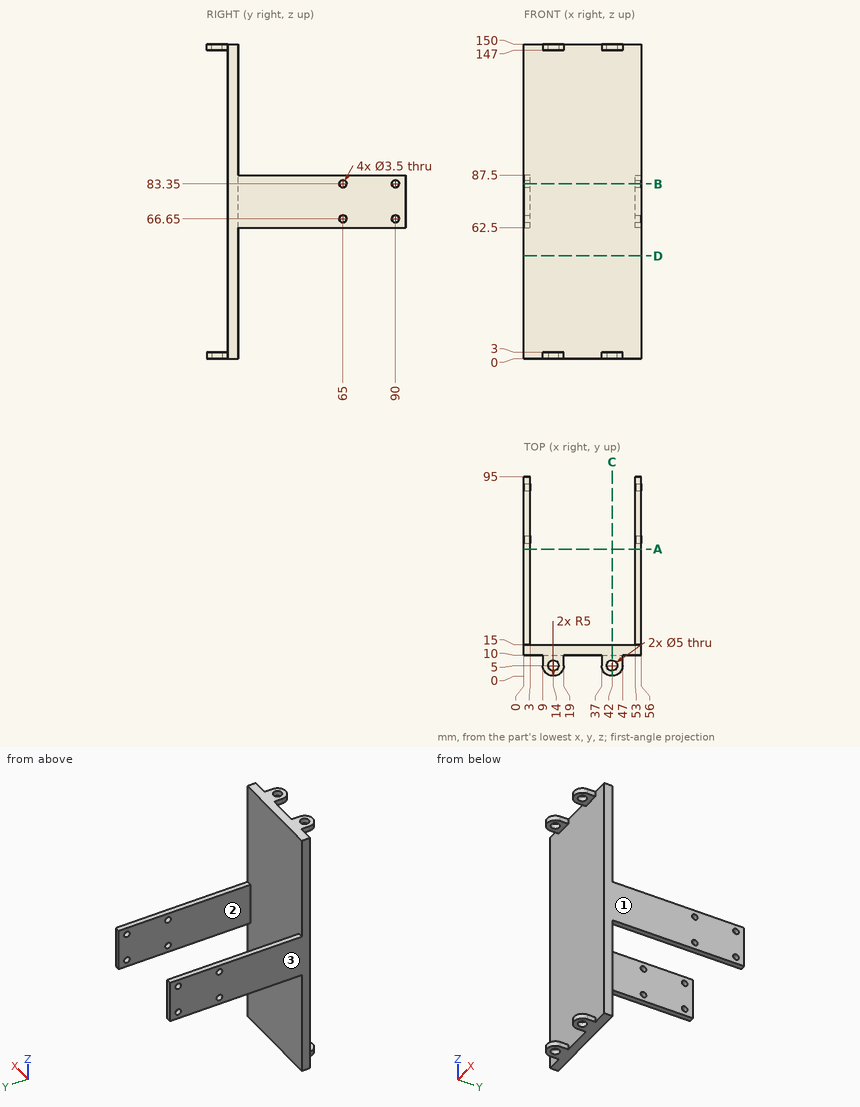
Design review of the part shown in the three views and the two pictorial views. Dimensions are in mm from the part's minimum x, y and z. Round coordinates to 2 decimals unless told otherwise and drop trailing zeros. Order: outer loops, then holes, each group sorted by start corner. A loop starts at its lowest first (then second) coordinate and runs counter-clockwise, first axis right, second up. Notation, with made-up numbers: (-14.5, 60) -> (35.5, 60) arc R32 cw to (35.5, 99) -> close; hole circle Ø7 at (-36, 58.25). An arc over 180 degrees is marked (long way). Write item = value, one per line. Start each with the question number.
1) Take a section at B-B on z = 83.35. State the section outline as (x, y) points, plus the area to 3 significant figures.
2) The part is to be moulded in two halves that separate along X. For the marked faces 1, 2 and 3, say which applies: +X half, -X half, draft (parallel to the pull), parting line (faces both ways), or undercut.
3) Take a section at D-D on z = 49. State the section outline as (x, y) points, plus the area to 3 significant figures.
4) Take a section at A-A on y = 60.5. State the section outline as (x, z) points, plus the area to 3 significant figures.
5) Insertion check: pin 1 (4 mm diameter, centred on x = 14, y = 5, fed in from +Z); pin 2 (4 mm diameter, centred on x = 24.5, z = 67, fed in from -Y); pin 3 (3 mm diameter, centred on x = 38, z = 108, fed in from +Y); pin 4 (1.5 mm diameter, centred on y = 8, z = 2, fed in from +X). Each pin has a flat end and moves straight along its axis. Give the tip position at first contact, or say it passes through.
6) To check wall thickness, follow line 1 (Z direction, x = 55, y = 65); line 2 (Y direction, x = 0.9, z = 83.35); line 3 (X direction, y = 44, z = 73). State the ranges of each line that lie inside material, in increasing order. Write a range as from..to.
7) Take a section at C-C on x = 42. State the section outline as (y, z) points.
Verdict:
q1.outline = (0, 10) -> (56, 10) -> (56, 63.25) -> (53, 63.25) -> (53, 15) -> (3, 15) -> (3, 63.25) -> (0, 63.25) -> close; (0, 66.75) -> (3, 66.75) -> (3, 88.25) -> (0, 88.25) -> close; (0, 91.75) -> (3, 91.75) -> (3, 95) -> (0, 95) -> close; (53, 66.75) -> (56, 66.75) -> (56, 88.25) -> (53, 88.25) -> close; (53, 91.75) -> (56, 91.75) -> (56, 95) -> (53, 95) -> close
q1.area = 718 mm2
q2.face_1 = +X half
q2.face_2 = undercut
q2.face_3 = -X half
q3.outline = (0, 10) -> (56, 10) -> (56, 15) -> (0, 15) -> close
q3.area = 280 mm2
q4.outline = (0, 62.5) -> (3, 62.5) -> (3, 87.5) -> (0, 87.5) -> close; (53, 62.5) -> (56, 62.5) -> (56, 87.5) -> (53, 87.5) -> close
q4.area = 150 mm2
q5.pin_1 = through
q5.pin_2 = 10
q5.pin_3 = 15
q5.pin_4 = 47
q6.line_1 = 62.5..64.9, 68.4..81.6, 85.1..87.5
q6.line_2 = 10..63.25, 66.75..88.25, 91.75..95
q6.line_3 = 0..3, 53..56
q7.outline = (0, 0) -> (2.5, 0) -> (2.5, 3) -> (0, 3) -> close; (0, 147) -> (2.5, 147) -> (2.5, 150) -> (0, 150) -> close; (7.5, 0) -> (15, 0) -> (15, 150) -> (7.5, 150) -> (7.5, 147) -> (10, 147) -> (10, 3) -> (7.5, 3) -> close
